The model under review builds one solid part; all positions refer to its coordinate system, in mm. Face numbers are marked on the shaded views. A direction names the side the tool comes from. Coordinates: 2 decimals unless noted, no trailing zeros. Order: outer loops, then holes, each group sorted by start corner. A loop starts at its lowest first (then second) coordinate and runs counter-clockwise, first axis right, second up. Notation, with made-up numbers: M 74,1 L 107,1 A19 cw 107,30 Z; hole C -17.5,4.25 d2. An arc over 180 degrees is marked long. Write each question's results on one line, items separated by ' | '.
Autodesk Inventor part; units mm, degrees
ref_plane "YZ Plane" through (0, 0, 0) normal (1, 0, 0) x (0, 1, 0)
ref_plane "XZ Plane" through (0, 0, 0) normal (0, 1, 0) x (-1, 0, 0)
ref_plane "XY Plane" through (0, 0, 0) normal (0, 0, 1) x (1, 0, 0)
sketch "Sketch1" plane through (0, 0, 0) normal (0, 0, 1) x (1, 0, 0)
  circle A0 centre (0, 0) radius 44.45
  circle A1 centre (-27.4963, 15.875) radius 6.35
  circle A2 centre (27.4963, 15.875) radius 6.35
  circle A3 centre (0, -31.75) radius 6.35
  dimension "d1" = 88.9
  dimension "d7" = 12.7
  dimension "d8" = 12.7
  dimension "d9" = 12.7
extrude "Extrusion3" add sketch "Sketch1" along normal blind 6.35
sketch "Sketch2" plane through (0, 0, 6.35) normal (0, 0, 1) x (1, 0, 0)
  circle A0 centre (0, 0) radius 12.7
  circle A1 centre (0, 0) radius 17.4625
  dimension "d16" = 25.4
  dimension "d17" = 34.925
extrude "Extrusion4" add sketch "Sketch2" along normal blind 6.35
sketch "Sketch3" plane through (0, 0, 6.35) normal (0, 0, 1) x (1, 0, 0)
  circle A0 centre (0, 0) radius 12.7
  dimension "d20" = 25.4
extrude "Extrusion5" cut sketch "Sketch3" against normal through all
properties part number "Assignment 1.6 Circular Spacer"
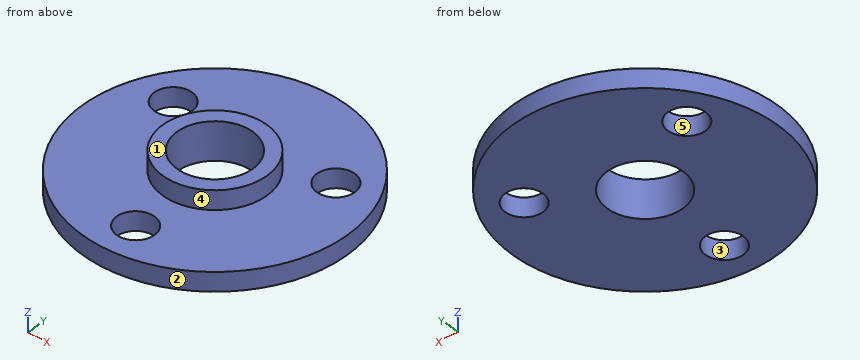
1) Take a section at C-C on x = -11. State the section outline as (y, z) points, plus the area to 3 significant figures.
Solutions:
outline: M -43.07,0 L -6.35,0 L -6.35,12.7 L -13.56,12.7 L -13.56,6.35 L -43.07,6.35 Z; M 6.35,0 L 43.07,0 L 43.07,6.35 L 13.56,6.35 L 13.56,12.7 L 6.35,12.7 Z | area: 558 mm2
2) Take a section at D-D on z = 10.5. State the section outline as (x, y) points (1 decimal), plus the area to 3 significant figures.
Solutions:
outline: C 0,0 d34.9; hole C 0,0 d25.4 | area: 451 mm2
3) For the marked faces 4 and 5, list the 3-axis set-ups (+Z, -Z, +X, -X, +Y, -Y) from which the entire face can be reached by the end or side of a thin tool; tool diameter is ignored.
Solutions:
face 4: +Z | face 5: +Z, -Z
4) Take a section at A-A on x = 0. State the section outline as (y, z) points, plus the area to 3 significant figures.
Solutions:
outline: M -44.45,0 L -38.1,0 L -38.1,6.35 L -44.45,6.35 Z; M -25.4,0 L -12.7,0 L -12.7,12.7 L -17.46,12.7 L -17.46,6.35 L -25.4,6.35 Z; M 12.7,0 L 44.45,0 L 44.45,6.35 L 17.46,6.35 L 17.46,12.7 L 12.7,12.7 Z | area: 383 mm2
5) The part is to be moulded in two halves that separate along X. For the marked faces 1, 2 and 3, say which applies: pulls with the +X half, pulls with the -X half, needs draft (parallel to the pull), parting line crosses it, or undercut.
Solutions:
face 1: needs draft | face 2: parting line crosses it | face 3: undercut
6) To check wall thickness, follow line 1 along Y through (x, z) = (0, 3); line 2 along Z through (x, y) = (-23.5, 25); line 3 along X through (y, z) = (-33.5, 1). State the ranges of each line that lie inside material, in increasing order.
Solutions:
line 1: -44.45 to -38.1, -25.4 to -12.7, 12.7 to 44.45 | line 2: 0 to 6.35 | line 3: -29.22 to -6.1, 6.1 to 29.22
7) For pin 1 (1.5 mm diameter, centred on y = 16, z = 7, fed in from -X); pin 2 (1.5 mm diameter, centred on x = 18.5, z = 5, fed in from +Y); pin 3 (6 mm diameter, centred on y = -30, z = 3.5, fed in from +X), all flat-tipped, find the tip position at first contact; note any pin that passes through.
Solutions:
pin 1: x = -41.61 | pin 2: y = 40.75 | pin 3: x = 35.31
8) Take a section at B-B on y = 0. State the section outline as (x, z) points, plus the area to 3 significant figures.
Solutions:
outline: M -44.45,0 L -12.7,0 L -12.7,12.7 L -17.46,12.7 L -17.46,6.35 L -44.45,6.35 Z; M 12.7,0 L 44.45,0 L 44.45,6.35 L 17.46,6.35 L 17.46,12.7 L 12.7,12.7 Z | area: 464 mm2
